Could you check a few things on this drawing? It's one solid part, dimensions in mm from its lowest x, y, z. A direction names the side the tool comes from. Round coordinates to 2 decimals unless told otherwise and drop trailing zeros. Write each loop counter-clockwise with the first axis right and the second up, starting at its lowest first coordinate (ties: lowest second). Pieces come first, ordered by that corner, then holes. Notation, with made-up numbers: (-36.75, 34) -> (-12.75, 34) arc R37 ccw to (-12.75, 73) -> close; hole circle Ø6 at (32.5, 26). An arc over 180 degrees is marked (long way). Answer in a Markdown table with one row per item. Add a question column.
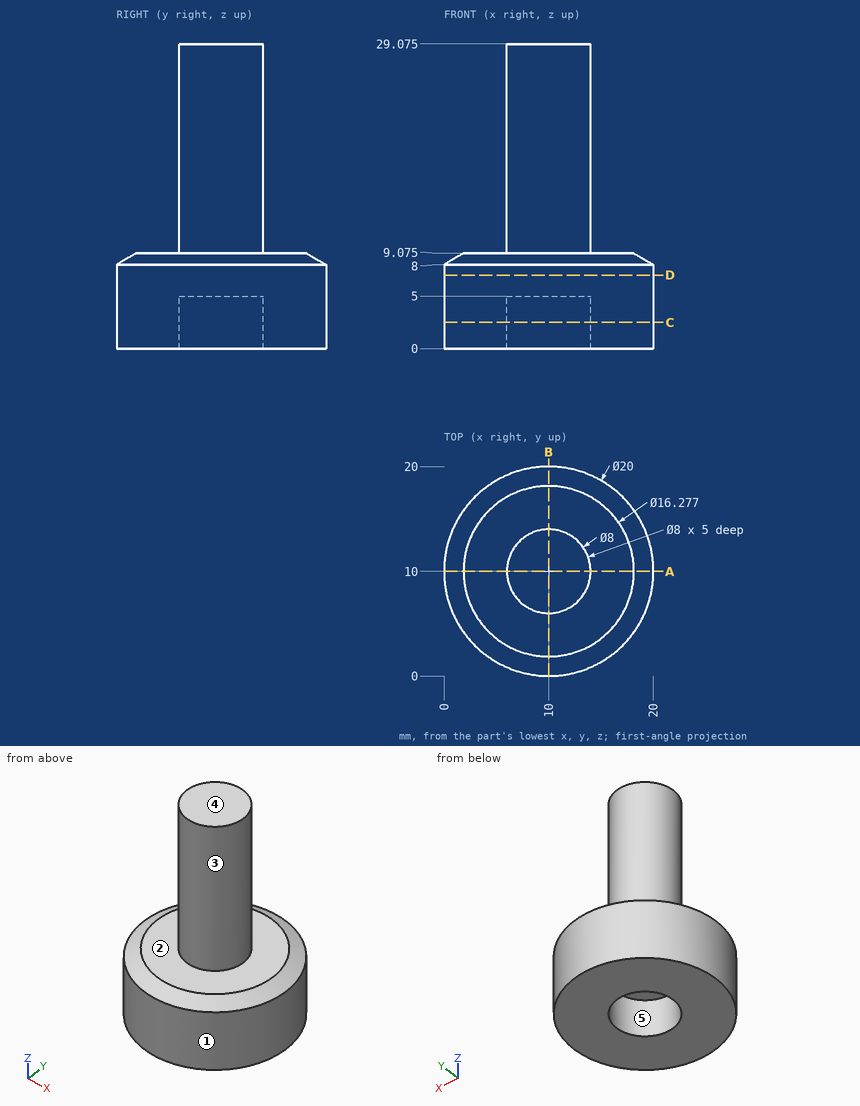
Item 1: If we section it at C-C on z = 2.5: Please give me the cut outline in (x, y).
Item 2: I need wall thicknesses on line 1 along X through (y, z) = (10, 3.6); line 2 along Z through (x, y) = (17.75, 7.5). Which ranges of each line are inside material? Lowest first, please. Write a range as from..to.
Item 3: For P1, Ø4, axis at x = 10, y = 9, coming from the -Z side; P2, Ø5, axis at y = 6.5, z = 6, coming from the -X side; P3, Ø1, axis at x = 7, z = 11, coming from the -Y side, each with a flat end and sliding along its axis, tell me the tip position at first contact or that it passes through.
Item 4: If we section it at A-A on y = 10: Please give me the cut outline in (x, z) (1 decimal).
Item 5: If we mould it in two halves opening along X, with no side actions, what happens to the marked faces 3, 4 and 5? For each: pulls with the +X half, pulls with the -X half, needs draft (parallel to the pull), parting line crosses it, or undercut.
Item 6: On a 3-axis mill with a long thin cutter (end or side, diameter ignored), from which of +Z, -Z, +X, -X, +Y, -Y can I reach the whole of each face in a straight line? I mean the marked faces 1 and 2. Say none if no direction works.
Item 7: If we section it at D-D on z = 7: Please give me the cut outline in (x, y).
Results list:
| question | item | result |
|---|---|---|
| 1 | outline | circle Ø20 at (10, 10); hole circle Ø8 at (10, 10) |
| 2 | line 1 | 0..6, 14..20 |
| 2 | line 2 | 0..9.07 |
| 3 | P1 | z = 5 |
| 3 | P2 | x = 0.05 |
| 3 | P3 | y = 6.88 |
| 4 | outline | (0, 0) -> (6, 0) -> (6, 5) -> (14, 5) -> (14, 0) -> (20, 0) -> (20, 8) -> (18.1, 9.1) -> (14, 9.1) -> (14, 29.1) -> (6, 29.1) -> (6, 9.1) -> (1.9, 9.1) -> (0, 8) -> close |
| 5 | face 3 | parting line crosses it |
| 5 | face 4 | needs draft |
| 5 | face 5 | undercut |
| 6 | face 1 | +Z, -Z |
| 6 | face 2 | +Z |
| 7 | outline | circle Ø20 at (10, 10) |
